Here's how the part is built. I have some questions about the finished solid (model axes, mm). Give positions to 0.01 mm unless a question says otherwise; leave off trailing zeros. Order: outer loops, then holes, each group sorted by start corner. A loop starts at its lowest first (then second) coordinate and runs counter-clockwise, first axis right, second up. Notation, with made-up numbers: M -4.75,53.25 L 39.25,53.25 A27 ccw 39.25,78.25 Z; hole C -9,-39 d11. An arc over 180 degrees is marked long. One line per item, written item: value. Start each with the question number.
from build123d import *

# Parameters (mm, degrees)
BOSS_EXTRUDE1_DEPTH     = 105
CUT_EXTRUDE1_DEPTH      = 50
CUT_EXTRUDE1_DEPTH_BACK = 50
SKETCH2_R               = 5


with BuildPart() as part:
    # Sketch1 → Boss-Extrude1 (new, symmetric)
    with BuildSketch(Plane.XY):
        Polygon((25, 5), (35, -5), (25, -5), (-25, -5), (-25, 5), align=None)
    extrude(amount=BOSS_EXTRUDE1_DEPTH, both=True)

    # Sketch2 → Cut-Extrude1 (cut, two sides: drawn at the far end of the back side and taken through both)
    with BuildSketch(Plane(origin=(0, 0, 0), x_dir=(1, 0, 0), z_dir=(0, 1, 0)).offset(-CUT_EXTRUDE1_DEPTH_BACK)):
        with Locations(Location((0, 50, 0), (0, 0, 180))):
            Circle(SKETCH2_R)
        with Locations(Location((0, -50, 0), (0, 0, 180))):
            Circle(SKETCH2_R)
    extrude(amount=CUT_EXTRUDE1_DEPTH + CUT_EXTRUDE1_DEPTH_BACK, mode=Mode.SUBTRACT)


solid = part.part
Item 1: I want a section at D-D on z = 91. Write out the boundary of the cut face in (x, y), plus the area to 3 significant figures.
Item 2: I want a section at A-A on x = 0. Write out the boundary of the cut face in (y, z), plus the area to 3 significant figures.
Item 3: I want a section at C-C on y = -0.25. Write out the boundary of the cut face in (x, z).
Item 4: We'd pull the mould along X, two halves only. Please class faces 1 (the face through (0.651, -0.07, 54.957)), 2 (the face through (0.651, -0.07, -45.043)), 3 (the face through (0, 5, 1)), 4 (the face through (30, 0, 1)): +X half, -X half, draft (parallel to the pull), parting line (faces both ways), or undercut.
Item 5: Will this pin go through, and if not, where does the flat tip stop? P1, Ø11.5, axis at x = 0, z = -50, coming from the +Y side.
Item 6: Please list where these lines run through material, in increasing order: probe 1 along Z at (x, y) = (0, -2.25); probe 2 along X at (y, z) = (-1.25, -50); probe 3 along X at (y, z) = (0.75, 50). Write a range as [from, to].
Item 7: I want a section at B-B on z = 50. Write out the boundary of the cut face in (x, y).
Answer below:
1. outline: M -25,-5 L 35,-5 L 25,5 L -25,5 Z
1. area: 550 mm²
2. outline: M -5,-105 L 5,-105 L 5,-55 L -5,-55 Z; M -5,-45 L 5,-45 L 5,45 L -5,45 Z; M -5,55 L 5,55 L 5,105 L -5,105 Z
2. area: 1,900 mm²
3. outline: M -25,-105 L 30.25,-105 L 30.25,105 L -25,105 Z; hole C 0,-50 d10; hole C 0,50 d10
4. face 1: undercut
4. face 2: undercut
4. face 3: draft
4. face 4: +X half
5. P1: stops at y = 5
6. probe 1: z = [-105, -55], [-45, 45], [55, 105]
6. probe 2: x = [-25, -5], [5, 31.25]
6. probe 3: x = [-25, -5], [5, 29.25]
7. outline: M -25,-5 L -5,-5 L -5,5 L -25,5 Z; M 5,-5 L 35,-5 L 25,5 L 5,5 Z
